For this review, use the dimensioned drawing (mm, ordinates from the lowest corner) and the shaded views. A direction names the side the tool comes from. Coordinates: 2 decimals unless noted, no trailing zeros. Loops run counter-clockwise (first coordinate to the right, second up) from the corner with the lowest first, then second, coordinate; pieces in that order, holes last. Notation, with made-up numbers: (46.25, -13.5) -> (92.25, -13.5) arc R25 ccw to (92.25, 14.5) -> close; hole circle Ø11 at (60, 71.25). An arc over 180 degrees is marked (long way). Use one line per item in the form item = value. Start each with the question number.
1. Consider section D-D (y = 61). State the section outline as (x, z) points (1 decimal).
2. The part is to be moulded in two halves that separate along X. For the marked faces 1, 2, 3 and 4, say which applies: released by +X, released by -X, zero draft, split by the parting line, or undercut.
3. For pin 1 (4 mm diameter, centred on x = 17, z = 10.5, fed in from +Y), flat-tipped, find the tip position at first contact; note if it passes through.
4. Consider section C-C (z = 18.5). State the section outline as (x, y) points (1 decimal), then the cut area to 3 significant figures.
5. Consider section B-B (y = 85). State the section outline as (x, z) points (1 decimal), then the cut area to 3 significant figures.
6. Wall thickness on line 1 (X direction, y = 64.5, z = 23.5) (1 decimal); line 2 (Y direction, x = 18.5, z = 16); line 3 (X direction, y = 94, z = 35): over which ranges is each line inside the solid? List them lowest first. Write a range as from..to.
7. Machinability: for the marked faces 5, 6 and 7, which of the approach directions +Z, -Z, +X, -X, +Y, -Y give a long, thin tool a straight path to every point of the face, cutting with its end or side? Answer none if there is none.
8. Consider section A-A (x = 41). State the section outline as (y, z) points.
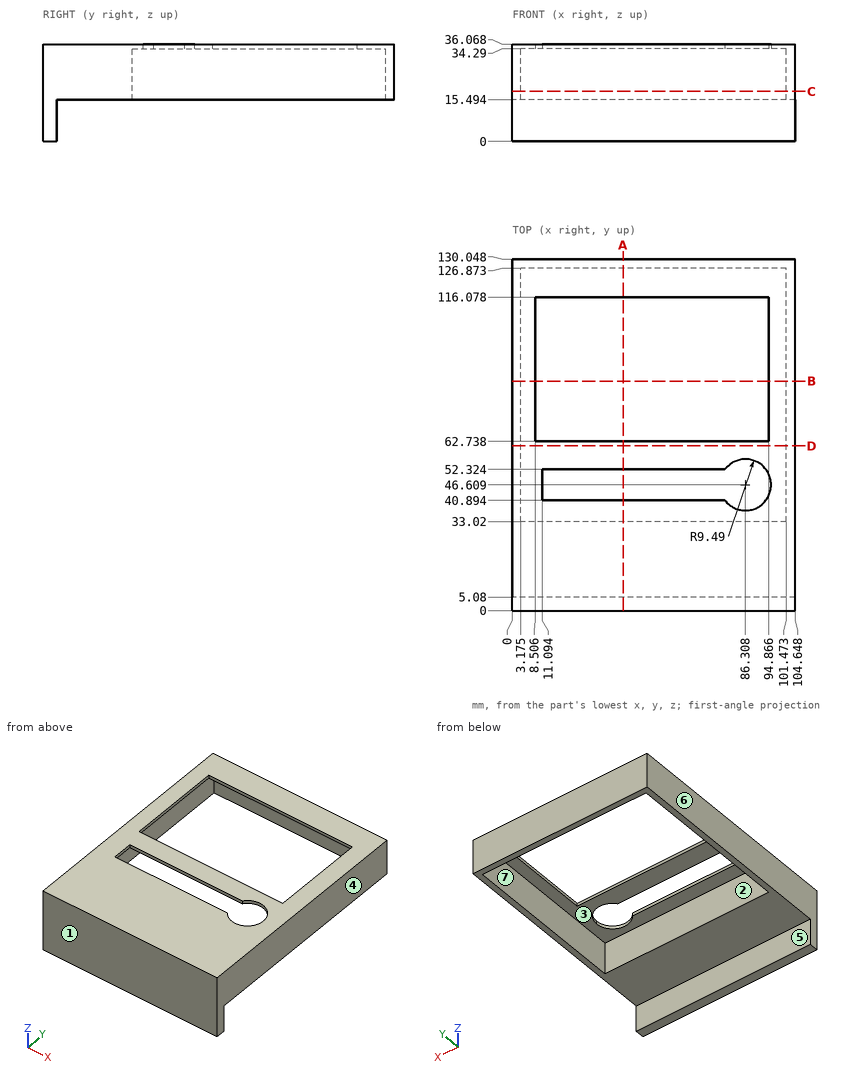
Geometry check:
q1.outline = (0, 15.5) -> (3.2, 15.5) -> (3.2, 34.3) -> (101.5, 34.3) -> (101.5, 15.5) -> (104.6, 15.5) -> (104.6, 36.1) -> (0, 36.1) -> close
q2.face_1 = zero draft
q2.face_2 = undercut
q2.face_3 = undercut
q2.face_4 = released by +X
q3.pin_1 = 5.08
q4.outline = (0, 0) -> (104.6, 0) -> (104.6, 130) -> (0, 130) -> close; hole (3.2, 33) -> (101.5, 33) -> (101.5, 126.9) -> (3.2, 126.9) -> close
q4.area = 4,380 mm²
q5.outline = (0, 15.5) -> (3.2, 15.5) -> (3.2, 34.3) -> (8.5, 34.3) -> (8.5, 36.1) -> (0, 36.1) -> close; (94.9, 34.3) -> (101.5, 34.3) -> (101.5, 15.5) -> (104.6, 15.5) -> (104.6, 36.1) -> (94.9, 36.1) -> close
q5.area = 152 mm²
q6.line_1 = 0..3.2, 101.5..104.6
q6.line_2 = 0..33.02, 126.87..130.05
q6.line_3 = 0..8.51, 94.87..104.65
q7.face_5 = -Z, +X, -X, +Y
q7.face_6 = +Z, -Z, -X, +Y, -Y
q7.face_7 = -Z
q8.outline = (0, 0) -> (5.08, 0) -> (5.08, 15.49) -> (33.02, 15.49) -> (33.02, 34.29) -> (40.89, 34.29) -> (40.89, 36.07) -> (0, 36.07) -> close; (52.32, 34.29) -> (62.74, 34.29) -> (62.74, 36.07) -> (52.32, 36.07) -> close; (116.08, 34.29) -> (126.87, 34.29) -> (126.87, 15.49) -> (130.05, 15.49) -> (130.05, 36.07) -> (116.08, 36.07) -> close
